Source: CAD feature listing. Evaluate the final solid. Frame: model axes, mm. Face numbers are marked on the shaded views. A direction names the side the tool comes from. Round coordinates to 2 decimals unless told otherwise and drop trailing zeros. Order: outer loops, then holes, each group sorted by start corner. A loop starts at its lowest first (then second) coordinate and runs counter-clockwise, first axis right, second up. Notation, with made-up numbers: M -25.75,-24 L 17.25,-24 A26 cw 17.25,9 Z; hole C 38,69.25 d4. An arc over 180 degrees is marked long. Use CSV: the item, a comma, the result in double quotes. Start each with the question number.
```python
from build123d import *

# Parameters (mm, degrees)
BOSS_EXTRUDE1_DEPTH = 70.45
SKETCH2_R           = 0.574746223
SKETCH2_R_2         = 0.572709313
BOSS_EXTRUDE2_DEPTH = 2


with BuildPart() as part:
    # Sketch1 → Boss-Extrude1 (new body)
    with BuildSketch(Plane(origin=(0, 0, 0), x_dir=(1, 0, 0), z_dir=(0, 1, 0))):
        with BuildLine():
            Line((-10.463385515, 13.437573917), (-10.463385515, 11.929541616))
            ThreePointArc((-10.463385515, 11.929541616), (-20.316677089, 0), (-10.463385515, -11.929541616))
            Line((-10.463385515, -11.929541616), (11.536614485, -11.929541616))
            ThreePointArc((11.536614485, -11.929541616), (21.38990606, 0), (11.536614485, 11.929541616))
            Line((11.536614485, 11.929541616), (5.132924913, 13.437573917))
            Line((5.132924913, 13.437573917), (-10.463385515, 13.437573917))
        make_face()
        with BuildLine():
            ThreePointArc((-10.463385515, -10.389541616), (-18.808385515, 0), (-10.463385515, 10.389541616))
            Line((-10.463385515, 10.389541616), (4.788760706, 10.389541616))
            Line((4.788760706, 10.389541616), (4.788760706, 11.929541616))
            Line((4.788760706, 11.929541616), (11.536614485, 10.389541616))
            ThreePointArc((11.536614485, 10.389541616), (19.881614485, 0), (11.536614485, -10.389541616))
            Line((11.536614485, -10.389541616), (-10.463385515, -10.389541616))
        make_face(mode=Mode.SUBTRACT)
    extrude(amount=BOSS_EXTRUDE1_DEPTH)

    # Sketch2 → Boss-Extrude2 (add)
    with BuildSketch(Plane.ZY.offset(10.463385515)):
        with Locations(Location((-12.681906896, 34.013885353, 0), (0, 0, 180))):
            Circle(SKETCH2_R)
        with Locations(Location((-12.681906896, 36.442241885, 0), (0, 0, 180))):
            Circle(SKETCH2_R_2)
    extrude(amount=BOSS_EXTRUDE2_DEPTH)


solid = part.part
```
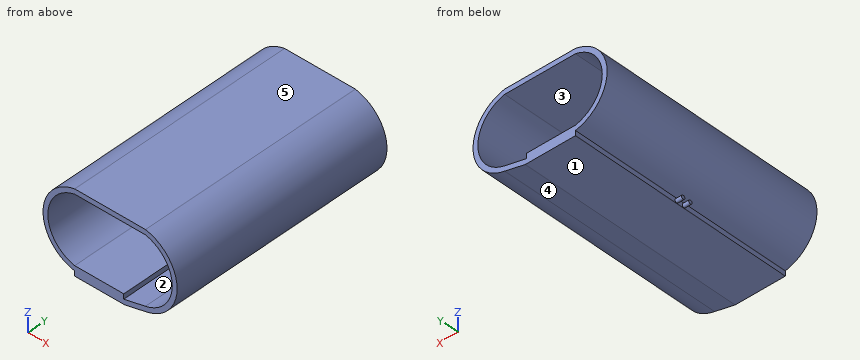
(1) Section A-A on x = -4. Return loops of the section in (y, z), plus the area to 3 significant figures.
(2) Draft query along X for the marked faces 3, 4 and 5. Return one class per face: pulls with the +X half, pulls with the -X half, needs draft (parallel to the pull), parting line crosses it, or undercut.
(3) Reachability of the marked faces 1 and 2 from +Z, -Z, +X, -X, +Y, -Y: full face, straight path, thin tool, end or side. Return the list, or none.
(4) Section D-D on x = -11.5. Return loops of the section in (y, z), plus the area to 3 significant figures.
(5) Line query: line 1 along X through (y, z) = (4, -0.5); line 2 along Z through (x, y) = (-6, 24); line 3 along X through (y, z) = (23.5, 1.75). Output: solid intervals per line, ascending.
(6) Contact query for flat-ended pins moving along their axis: P1, Ø1.5, axis at y = 46.5, z = 6, coming from the +X side; P2, Ø1.5, axis at x = 17, y = 30, coming from the -Z side; P3, Ø5, axis at y = 19.5, z = -4.5, coming from the -X side; P4, Ø8, axis at x = 12.5, z = 1.5, coming from the -Y side. Output: stop coordinate, or through.
(7) Section C-C on z = 1.5. Return loops of the section in (x, y), plus the area to 3 significant figures.
(8) Section B-B on y = 10. Return loops of the section in (x, z).
Results below:
1,outline,"M 0,-13.44 L 70.45,-13.44 L 70.45,-10.39 L 0,-10.39 Z; M 0,10.39 L 70.45,10.39 L 70.45,11.93 L 0,11.93 Z"
1,area,"323 mm2"
2,face 3,"undercut"
2,face 4,"pulls with the +X half"
2,face 5,"needs draft"
3,face 1,"-Z, +X, -X, +Y, -Y"
3,face 2,"+Y, -Y"
4,outline,"M 0,-11.68 L 70.45,-11.68 L 70.45,-10.1 L 0,-10.1 Z; M 0,10.1 L 70.45,10.1 L 70.45,11.68 L 0,11.68 Z; C 34.01,-12.68 d1.15; C 36.44,-12.68 d1.15"
4,area,"224 mm2"
5,line 1,"x = -20.31 to -18.8, 19.87 to 21.38"
5,line 2,"z = -13.44 to -10.39, 10.39 to 11.93"
5,line 3,"x = -20.19 to -18.66, 19.74 to 21.26"
6,P1,"stops at x = 20.2"
6,P2,"stops at z = -9.92"
6,P3,"stops at x = -20.15"
6,P4,"passes through"
7,outline,"M -20.22,0 L -18.7,0 L -18.7,70.45 L -20.22,70.45 Z; M 19.78,0 L 21.3,0 L 21.3,70.45 L 19.78,70.45 Z"
7,area,"214 mm2"
8,outline,"M -10.46,-13.44 L 5.13,-13.44 L 11.54,-11.93 A12.15 ccw 11.54,11.93 L -10.46,11.93 A12.15 ccw -10.46,-11.93 Z; hole M -10.46,-10.39 L 4.79,-10.39 L 4.79,-11.93 L 11.54,-10.39 A10.64 ccw 11.54,10.39 L -10.46,10.39 A10.64 ccw Z"
